Autodesk Inventor part; units mm, degrees
ref_plane "YZ Plane" through (0, 0, 0) normal (1, 0, 0) x (0, 1, 0)
ref_plane "XZ Plane" through (0, 0, 0) normal (0, 1, 0) x (-1, 0, 0)
ref_plane "XY Plane" through (0, 0, 0) normal (0, 0, 1) x (1, 0, 0)
sketch "Sketch1" plane through (0, 0, 0) normal (1, 0, 0) x (0, 1, 0)
  line L0 (0, 0) -> (25.4, 0)
  line L1 (25.4, 0) -> (25.4, -25.4)
  line L2 (25.4, -25.4) -> (0, -25.4)
  line L3 (0, -25.4) -> (0, 0)
  line L4 (0, 0) -> (3.175, 0)
  line L5 (0, -3.175) -> (0, 0)
  line L6 (3.175, -3.175) -> (22.225, -3.175)
  line L7 (22.225, -3.175) -> (22.225, -22.225)
  line L8 (22.225, -22.225) -> (3.175, -22.225)
  line L9 (3.175, -22.225) -> (3.175, -3.175)
  dimension "d0" = 25.4
  dimension "d1" = 25.4
  dimension "d6" = 19.05
  dimension "d7" = 19.05
extrude "Extrusion1" add sketch "Sketch1" along normal blind 101.6 contours L0 L1 L2 L3 | L6 L7 L8 L9
sketch "Sketch2" plane through (101.6, 0, 0) normal (1, 0, 0) x (0, 0, -1)
  line L0 (22.733, 22.225) -> (22.733, 22.733)
  line L1 (22.733, 22.733) -> (22.225, 22.733)
  line L2 (2.667, 3.175) -> (2.667, 2.667)
  line L3 (2.667, 2.667) -> (3.175, 2.667)
  line L4 (2.667, 2.667) -> (22.733, 2.667)
  line L5 (22.733, 2.667) -> (22.733, 22.733)
  line L6 (22.733, 22.733) -> (2.667, 22.733)
  line L7 (2.667, 22.733) -> (2.667, 2.667)
  point P0 (0, 0)
extrude "Extrusion2" cut sketch "Sketch2" against normal blind 50.8
sketch "Sketch3" plane through (0, 0, 0) normal (-1, 0, 0) x (0, 0, 1)
  line L0 (-25.4, 0) -> (-21.6315, 0)
  line L1 (-21.6315, 3.81) -> (-17.78, 3.81)
  line L2 (-21.6315, 7.62) -> (-21.6315, 3.81)
  line L3 (-3.81, 21.59) -> (-7.62, 21.59)
  line L4 (-3.81, 17.78) -> (-3.81, 21.59)
  line L5 (-21.6315, 3.81) -> (-3.81, 3.81)
  line L6 (-3.81, 3.81) -> (-3.81, 21.59)
  line L7 (-3.81, 21.59) -> (-21.6315, 21.59)
  line L8 (-21.6315, 21.59) -> (-21.6315, 3.81)
  line L9 (-17.8215, 7.6198) -> (-7.62, 7.6198)
  line L10 (-7.62, 7.6198) -> (-7.62, 17.78)
  line L11 (-7.62, 17.78) -> (-17.8215, 17.78)
  line L12 (-17.8215, 17.78) -> (-17.8215, 7.6198)
  point P0 (0, 25.4)
extrude "Extrusion3" add sketch "Sketch3" along normal blind 38.1
properties part number "Right Side Piece"
Check sheet for the modelled part. Datum: model origin and axes. Units: mm. A direction names the side the tool comes from. Round coordinates to 2 decimals unless told otherwise and drop trailing zeros. Order: outer loops, then holes, each group sorted by start corner. A loop starts at its lowest first (then second) coordinate and runs counter-clockwise, first axis right, second up. Notation, with made-up numbers: M 38,25.5 L 82,25.5 A14 cw 82,35.5 Z; hole C 59,-2.75 d9. An arc over 180 degrees is marked long. One line per item, written item: value. Start each with the question number.
1. Gauge pin test, flat ends, axial feed: P1, Ø10, axis at y = 12.5, z = -12, coming from the +X side; P2, Ø10, axis at x = 69, z = -12.5, coming from the -Y side; P3, Ø3, axis at x = -21, y = 12.5, coming from the +Z side; P4, Ø5, axis at x = -24, y = 10.5, coming from the -Z side. Record the tip position at first contact, or that the pin passes through.
2. Section check C-C on z = -19.25. Enter the section's corners in (x, y), and give its area (3 significant figures).
3. Section check A-A on x = 52.5. Enter the section's corners in (y, z).
4. Section check D-D on z = -11.5. Enter the section's corners in (x, y).
5. Release check for a two-part mould opening along Y. For faces 1 (the flat face through (77, 22.733, -13)), 2 (the flat face through (50, 25.4, -13)), 3 (the flat face through (-38.1, 19, -13)) record: released by +Y, released by -Y, zero draft, split by the parting line, or undercut.
6. Section check B-B on y = 5. Enter the section's corners in (x, z), and give its area (3 significant figures).
7. Scan lines: line 1 along Z through (x, y) = (-8.5, 15.25); line 2 along Y through (x, z) = (-12.5, -8); line 3 along Y through (x, z) = (69.5, -3.5). Record each from-to range of solid material in increasing order.
8. Access from +Z, -Z, +X, -X, +Y, -Y to the whole of each face (thin tool, end or side, straight path). Record for faces 4 (the flat face through (77, 2.667, -13)), 5 (the flat face through (-19, 13, -3.81)), 6 (the flat face through (-19, 21.59, -13)), 7 (the flat face through (-19, 17.78, -13)), 8 (the flat face through (-19, 13, -21.632)).
Results found:
1. P1: x = 50.8
1. P2: y = 0
1. P3: z = -3.81
1. P4: z = -21.63
2. outline: M -38.1,3.81 L 0,3.81 L 0,0 L 101.6,0 L 101.6,2.67 L 50.8,2.67 L 50.8,22.73 L 101.6,22.73 L 101.6,25.4 L 0,25.4 L 0,21.59 L -38.1,21.59 Z
2. area: 2,240 mm^2
3. outline: M 0,-25.4 L 25.4,-25.4 L 25.4,0 L 0,0 Z; hole M 2.67,-22.73 L 22.73,-22.73 L 22.73,-2.67 L 2.67,-2.67 Z
4. outline: M -38.1,3.81 L 0,3.81 L 0,0 L 101.6,0 L 101.6,2.67 L 50.8,2.67 L 50.8,22.73 L 101.6,22.73 L 101.6,25.4 L 0,25.4 L 0,21.59 L -38.1,21.59 L -38.1,17.78 L 0,17.78 L 0,7.62 L -38.1,7.62 Z
5. face 1: undercut
5. face 2: released by +Y
5. face 3: zero draft
6. outline: M -38.1,-21.63 L 0,-21.63 L 0,-25.4 L 101.6,-25.4 L 101.6,-22.73 L 50.8,-22.73 L 50.8,-2.67 L 101.6,-2.67 L 101.6,0 L 0,0 L 0,-3.81 L -38.1,-3.81 Z
6. area: 2,240 mm^2
7. line 1: -21.63 to -17.82, -7.62 to -3.81
7. line 2: 3.81 to 7.62, 17.78 to 21.59
7. line 3: 0 to 2.67, 22.73 to 25.4
8. face 4: +X
8. face 5: +Z, -X, +Y, -Y
8. face 6: +Z, -Z, -X, +Y
8. face 7: -X
8. face 8: -Z, -X, +Y, -Y
